Verification items for this drawing (mm, ordinates from the low corner). Round coordinates to 2 decimals unless told otherwise and drop trailing zeros. Order: outer loops, then holes, each group sorted by start corner. A loop starts at its lowest first (then second) coordinate and runs counter-clockwise, first axis right, second up. Notation, with made-up numbers: (-18, 23.5) - (18, 23.5) arc R16 cw to (18, 42.5) - close; hole circle Ø8 at (8.5, 59). An arc over 180 degrees is marked (long way). Use a Markdown table: item, result. Add a question column.
(1) Gauge pin test, flat ends, axial feed: P1, Ø1, axis at x = 207, z = 68, coming from the +Y side (3 decimals); P2, Ø0.6, axis at x = 1, y = 1, coming from the -Z side; P3, Ø0.6, axis at y = 3, z = 49, coming from the +X side (3 decimals). Record the tip position at first contact, or that the pin passes through.
(2) Thickness scan on line 1 along X through (y, z) = (0.7, 31) (3 decimals); line 2 along X through (y, z) = (3.2, 101.5) (3 decimals). Record the ranges inside material, lowest first. Write a range as [from, to].
(3) Section check A-A on z = 108. Record the boundary of the cut face in (x, y) (3 decimals).
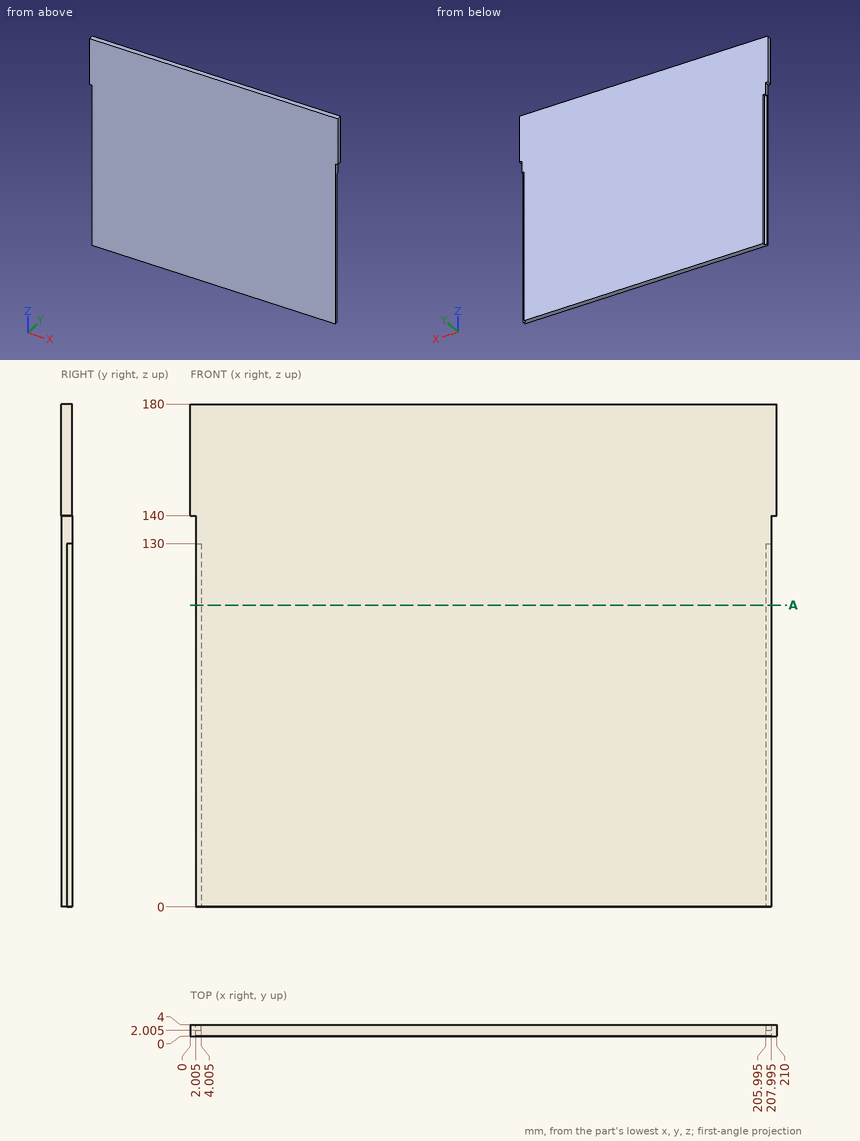
Check sheet entries:
| question | item | result |
|---|---|---|
| 1 | P1 | stops at y = 2.005 |
| 1 | P2 | stops at z = 140 |
| 1 | P3 | stops at x = 205.995 |
| 2 | line 1 | x = [2.005, 207.995] |
| 2 | line 2 | x = [4.005, 205.995] |
| 3 | outline | (2.005, 0) - (207.995, 0) - (207.995, 2.005) - (205.995, 2.005) - (205.995, 4) - (4.005, 4) - (4.005, 2.005) - (2.005, 2.005) - close |
